Answer from the drawing. Dimensions are ordinates in mm from the lowest x, y and z of the part. Coordinates: 2 decimals unless noted, no trailing zeros. Loops run counter-clockwise (first coordinate to the right, second up) from the corner with the lowest first, then second, coordinate; pieces in that order, holes last. Notation, with made-up numbers: M 27,-4 L 72,-4 A10 ccw 72,11 Z; hole C 32,58.5 d5. An arc over 180 degrees is marked long. Answer as CSV lines item,"result". Start each with the question number.
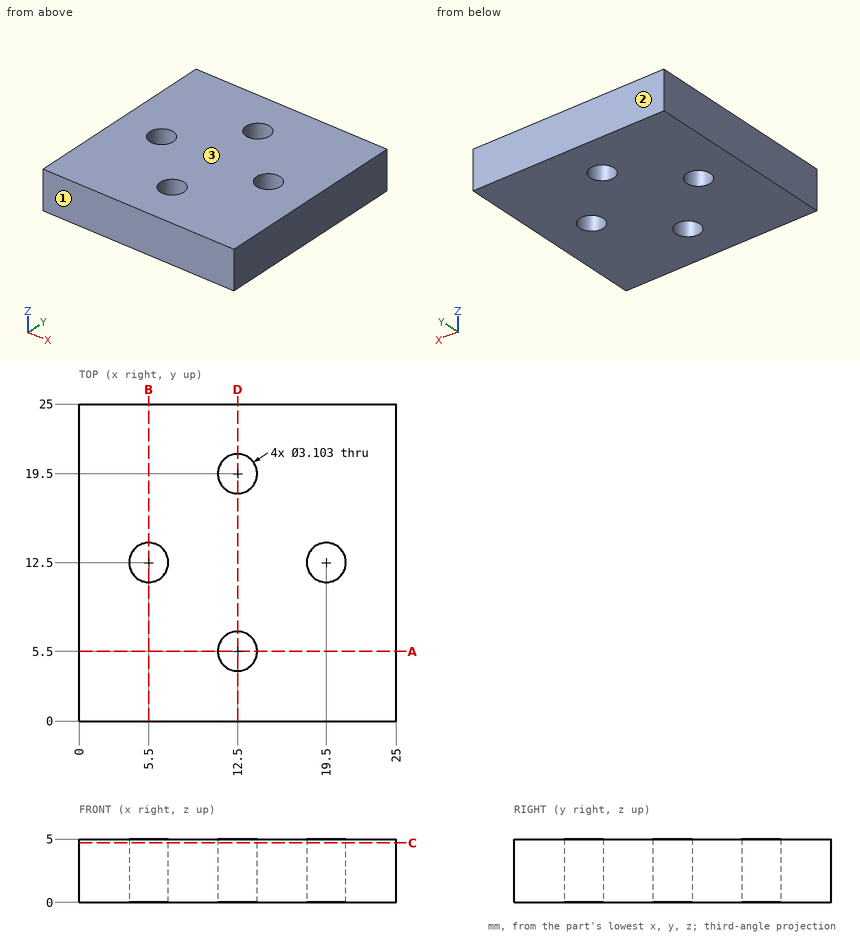
Item 1: Section D-D on x = 12.5 is taken. Determine the outline of the cut face in (y, z), then the cut area to 3 significant figures.
Item 2: Section A-A on y = 5.5 is taken. Determine the outline of the cut face in (x, z), then the cut area to 3 significant figures.
Item 3: Section C-C on z = 4.7 is taken. Determine the outline of the cut face in (x, y).
Item 4: For a pull along Y with two mould halves and no side action, classify the marked faces 1, 2 and 3 as pulls with the +Y half, pulls with the -Y half, needs draft (parallel to the pull), parting line crosses it, or undercut.
Item 5: Consider line 1 (Y direction, x = 12.5, z = 2.75); line 2 (Y direction, x = 5.5, z = 2.5); line 3 (Y direction, x = 18.75, z = 1.2). Determine where each line is inside the solid, lowest interval first.
Results are:
1,outline,"M 0,0 L 3.95,0 L 3.95,5 L 0,5 Z; M 7.05,0 L 17.95,0 L 17.95,5 L 7.05,5 Z; M 21.05,0 L 25,0 L 25,5 L 21.05,5 Z"
1,area,"94.0 mm²"
2,outline,"M 0,0 L 10.95,0 L 10.95,5 L 0,5 Z; M 14.05,0 L 25,0 L 25,5 L 14.05,5 Z"
2,area,"109 mm²"
3,outline,"M 0,0 L 25,0 L 25,25 L 0,25 Z; hole C 5.5,12.5 d3.1; hole C 12.5,5.5 d3.1; hole C 12.5,19.5 d3.1; hole C 19.5,12.5 d3.1"
4,face 1,"pulls with the -Y half"
4,face 2,"pulls with the +Y half"
4,face 3,"needs draft"
5,line 1,"0 to 3.95, 7.05 to 17.95, 21.05 to 25"
5,line 2,"0 to 10.95, 14.05 to 25"
5,line 3,"0 to 11.14, 13.86 to 25"
